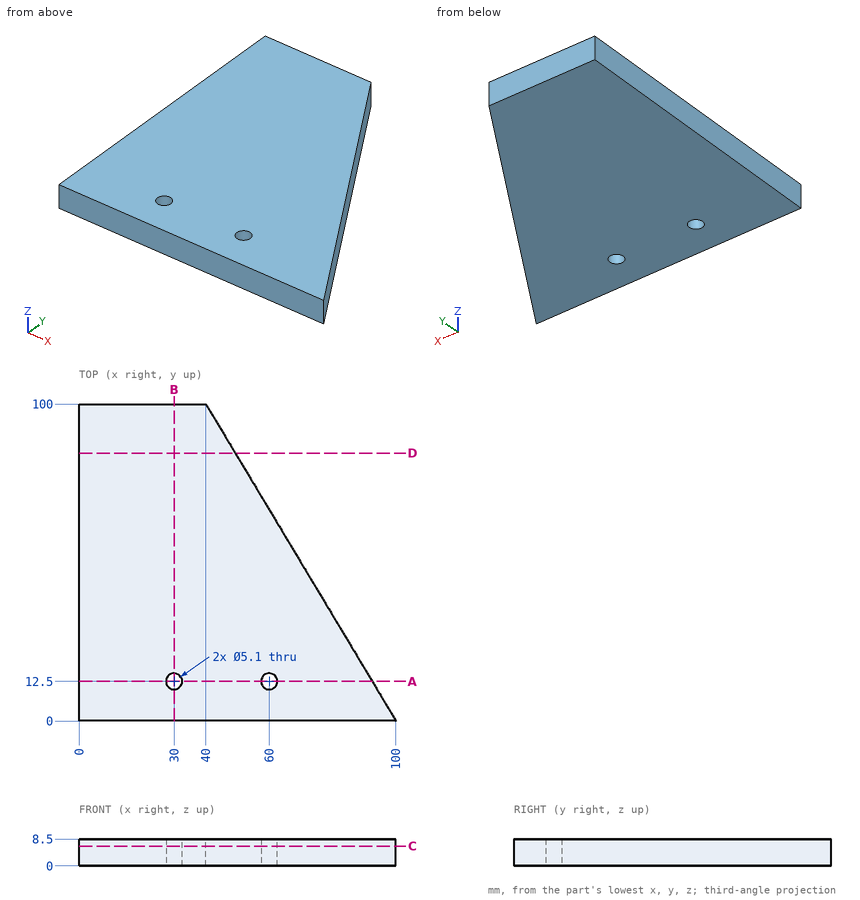
The figure shows three views and two pictorial views of one solid part (mm, origin at its lowest corner). Answer the questions. Give positions to 0.01 mm unless a question says otherwise; leave off trailing zeros. Write each loop counter-clockwise with the first axis right and the second up, starting at its lowest first coordinate (ties: lowest second). Pieces come first, ordered by that corner, then holes. Notation, with made-up numbers: (20.25, -11) -> (43.25, -11) arc R24 cw to (43.25, 20) -> close; hole circle Ø7 at (-36.5, 79.25). An arc over 180 degrees is marked (long way). Answer as a JSON object with one key per item and string values.
1) Section C-C on z = 6.25 is taken. Write down the section's boundary in (x, y).
Findings below:
{"outline": "(0, 0) -> (100, 0) -> (40, 100) -> (0, 100) -> close; hole circle Ø5.1 at (30, 12.5); hole circle Ø5.1 at (60, 12.5)"}
2) Straight lines are drawn through the part: probe 1 along Y at (x, z) = (30, 6.25); probe 2 along Y at (x, z) = (60, 4.75); probe 3 along Y at (x, z) = (46, 5). For each, find the intervals that lie inside material, in ascending order. Write a range as from..to.
Findings below:
{"probe 1": "y = 0..9.95, 15.05..100", "probe 2": "y = 0..9.95, 15.05..66.67", "probe 3": "y = 0..90"}
3) Section D-D on y = 84.5 is taken. Write down the section's boundary in (x, z), then the cut area to 3 significant figures.
Findings below:
{"outline": "(0, 0) -> (49.3, 0) -> (49.3, 8.5) -> (0, 8.5) -> close", "area": "419 mm^2"}
4) Section B-B on x = 30 is taken. Write down the section's boundary in (y, z), then the cut area to 3 significant figures.
Findings below:
{"outline": "(0, 0) -> (9.95, 0) -> (9.95, 8.5) -> (0, 8.5) -> close; (15.05, 0) -> (100, 0) -> (100, 8.5) -> (15.05, 8.5) -> close", "area": "807 mm^2"}
5) Section A-A on y = 12.5 is taken. Write down the section's boundary in (x, z).
Findings below:
{"outline": "(0, 0) -> (27.45, 0) -> (27.45, 8.5) -> (0, 8.5) -> close; (32.55, 0) -> (57.45, 0) -> (57.45, 8.5) -> (32.55, 8.5) -> close; (62.55, 0) -> (92.5, 0) -> (92.5, 8.5) -> (62.55, 8.5) -> close"}
6) Flat-ended cylindrical pins translate along their axes: pin 1 Ø3 at (y, z) = (79.5, 3) entering from +X; pin 2 Ø4.5 at (x, y) = (60, 12.5) entering from +Z. Find the tip coordinate at first contact, or state that the pin passes through.
Findings below:
{"pin 1": "stops at x = 53.2", "pin 2": "passes through"}
